Answer from the drawing. Dimensions are ordinates in mm from the lowest x, y and z of the part. Round coordinates to 2 decimals unless told otherwise and drop trailing zeros. Write each loop counter-clockwise with the first axis right and the second up, starting at its lowest first coordinate (ties: lowest second). Pieces come first, ordered by that corner, then holes. Notation, with made-up numbers: (56.5, 34.25) - (82.5, 34.25) arc R24 cw to (82.5, 56.25) - close; hole circle Ø2 at (53, -39.75). An arc over 180 degrees is marked (long way). Use a Markdown table: item, result. Add a question column.
1) Find the intervals of material crossed by probe 1 along Z at (x, y) = (68, 1.35); probe 2 along X at (y, z) = (2.45, 25.5); probe 3 along Z at (x, y) = (123.5, 2.3), in increasing order. Write a range as from..to.
2) Each of these flat-tipped pins is pushed along its axis until it touches: P1, Ø0.9, axis at y = 2, z = 1, coming from the +X side; P2, Ø1.5, axis at y = 1, z = 37, coming from the -X side; P3, Ø0.9, axis at x = 122, y = 1.5, coming from the -Z side. Where does it stop, or does it pass through?
3) A cutting plane is placed at C-C (z = 17). Give the vertices of the cut face in (x, y), then the cut area to 3 significant figures.
4) A cutting plane is placed at B-B (x = 71). Give the vertices of the cut face in (y, z), then the cut area to 3 significant figures.
5) A cutting plane is placed at A-A (z = 47). Give the vertices of the cut face in (x, y).
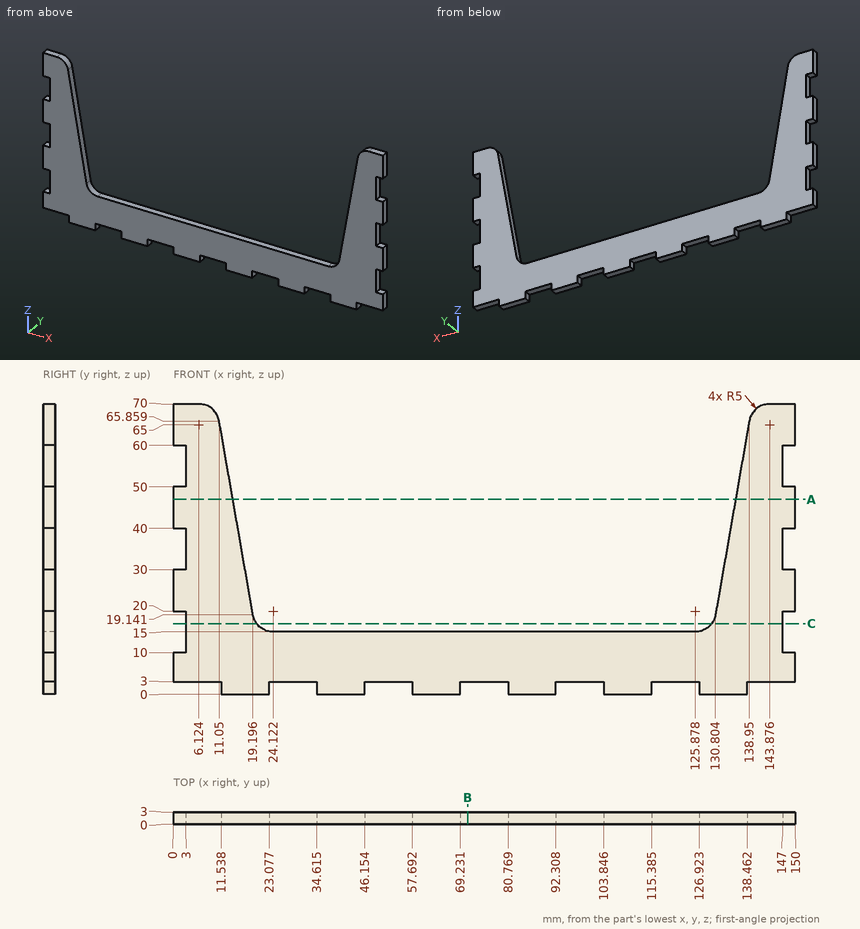
Entries:
| question | item | result |
|---|---|---|
| 1 | probe 1 | z = 0..15 |
| 1 | probe 2 | x = 0..18.09, 131.91..150 |
| 1 | probe 3 | z = 3..15 |
| 2 | P1 | stops at x = 138.46 |
| 2 | P2 | stops at x = 3 |
| 2 | P3 | stops at z = 3 |
| 3 | outline | (3, 0) - (20.12, 0) - (20.12, 3) - (3, 3) - close; (129.88, 0) - (147, 0) - (147, 3) - (129.88, 3) - close |
| 3 | area | 103 mm² |
| 4 | outline | (0, 3) - (3, 3) - (3, 15) - (0, 15) - close |
| 4 | area | 36.0 mm² |
| 5 | outline | (0, 0) - (14.34, 0) - (14.34, 3) - (0, 3) - close; (135.66, 0) - (150, 0) - (150, 3) - (135.66, 3) - close |
